The figure shows three views and two pictorial views of one solid part (mm, origin at its lowest corner). Answer the questions. A direction names the side the tool comes from. Round coordinates to 2 decimals unless told otherwise and drop trailing zeros. Write each loop counter-clockwise with the first axis right and the second up, starting at its lowest first coordinate (ties: lowest second). Pieces come first, ordered by that corner, then holes. Notation, with made-up numbers: (-36, 62.5) - (-16, 62.5) arc R11 cw to (-16, 67.5) - close; hole circle Ø2 at (85.5, 82.25). An arc over 180 degrees is marked (long way). Answer as CSV lines item,"result". Start each with the question number.
Item 1: Flat-ended cylindrical pins translate along their axes: pin 1 (1 mm diameter, centred on y = 14, z = 8, fed in from +X); pin 2 (1 mm diameter, centred on y = 2, z = 9, fed in from +X); pin 3 (1.5 mm diameter, centred on x = 2, y = 10, fed in from +Z). Find the tip coordinate at first contact, or state that the pin passes through.
Item 2: A cutting plane is placed at C-C on z = 9. Determine the outline of the cut face in (x, y), and give its area (3 significant figures).
Item 3: A cutting plane is placed at B-B on y = 12.75. Determine the outline of the cut face in (x, z), and give its area (3 significant figures).
Item 4: Straight lines are drawn through the part: line 1 along Y through (x, z) = (11, 4.25); line 2 along X through (y, z) = (11.25, 1.5); line 3 along Z through (x, y) = (1.75, 2.5). For each, find the intervals that lie inside material, in ascending order. Write a range as [from, to].
Item 5: A cutting plane is placed at A-A on z = 5. Determine the outline of the cut face in (x, y), and give its area (3 significant figures).
Item 6: Which of the six approach directions +Z, -Z, +X, -X, +Y, -Y give full straight-line access (tool end or side, diameter ignored) to the marked faces 1, 2 and 3?
Item 7: A cutting plane is placed at D-D on y = 4. Determine the outline of the cut face in (x, z), and give its area (3 significant figures).
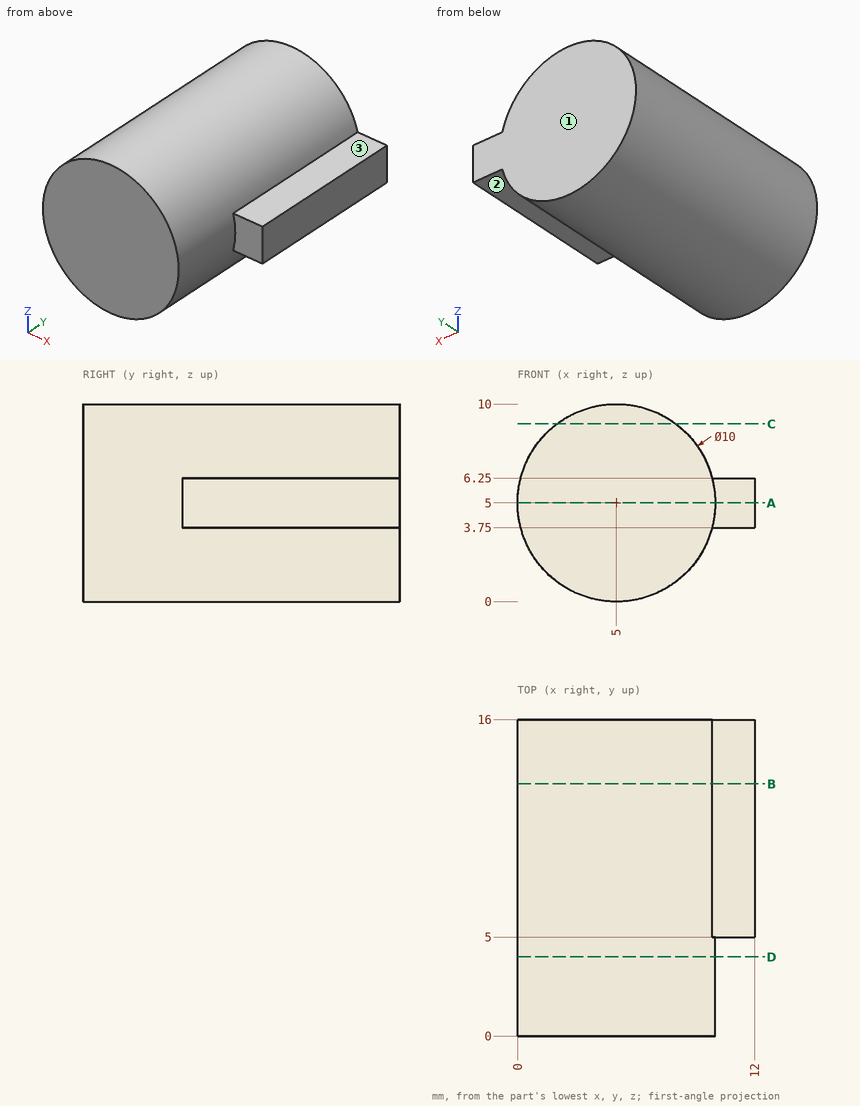
Geometry says:
1,pin 1,"stops at x = 9.33"
1,pin 2,"stops at x = 8.57"
1,pin 3,"stops at z = 9.47"
2,outline,"(2, 0) - (8, 0) - (8, 16) - (2, 16) - close"
2,area,"96.0 mm^2"
3,outline,"(9.84, 3.75) - (12, 3.75) - (12, 6.25) - (9.84, 6.25) arc R5 ccw (long way) to start"
3,area,"83.7 mm^2"
4,line 1,"y = [5, 16]"
4,line 2,"x = [1.43, 8.57]"
4,line 3,"z = [1.2, 8.8]"
5,outline,"(0, 0) - (10, 0) - (10, 5) - (12, 5) - (12, 16) - (0, 16) - close"
5,area,"182 mm^2"
6,face 1,"+Z, -Z, +X, -X, +Y"
6,face 2,"-Z, +X, +Y, -Y"
6,face 3,"+Z, +X, +Y, -Y"
7,outline,"circle Ø10 at (5, 5)"
7,area,"78.5 mm^2"
